```python
from build123d import *

# Parameters (mm, degrees)
SKETCH1_W           = 128
SKETCH1_H           = 73
SKETCH1_W_2         = 120
SKETCH1_H_2         = 65
BOSS_EXTRUDE1_DEPTH = 41
SKETCH1_3_W         = 128
SKETCH1_3_H         = 73
BOSS_EXTRUDE2_DEPTH = 4
SKETCH3_R           = 10.16
CUT_EXTRUDE1_DEPTH  = 4
SKETCH5_W           = 6
SKETCH5_H           = 65
BOSS_EXTRUDE3_DEPTH = 32
BOSS_EXTRUDE4_DEPTH = 32
CUT_EXTRUDE2_DEPTH  = 10


with BuildPart() as part:
    # Sketch1 → Boss-Extrude1 (new body)
    with BuildSketch(Plane(origin=(0, 0, 0), x_dir=(1, 0, 0), z_dir=(0, 1, 0))):
        Rectangle(SKETCH1_W, SKETCH1_H)
        Rectangle(SKETCH1_W_2, SKETCH1_H_2, mode=Mode.SUBTRACT)
    extrude(amount=BOSS_EXTRUDE1_DEPTH)

    # Sketch1<3> → Boss-Extrude2 (add)
    with BuildSketch(Plane(origin=(0, 0, 0), x_dir=(1, 0, 0), z_dir=(0, 1, 0))):
        Rectangle(SKETCH1_3_W, SKETCH1_3_H)
    extrude(amount=-BOSS_EXTRUDE2_DEPTH)

    # Sketch3 → Cut-Extrude1 (cut)
    with BuildSketch(Plane.XY.offset(36.5)):
        with Locations((-44, 21)):
            Circle(SKETCH3_R)
    extrude(amount=-CUT_EXTRUDE1_DEPTH, mode=Mode.SUBTRACT)

    # Sketch5 → Boss-Extrude3 (add)
    with BuildSketch(Plane(origin=(0, 0, 0), x_dir=(1, 0, 0), z_dir=(0, 1, 0))):
        with Locations((-11.5, 0)):
            Rectangle(SKETCH5_W, SKETCH5_H)
    extrude(amount=BOSS_EXTRUDE3_DEPTH)

    # Sketch8 → Boss-Extrude4 (add)
    with BuildSketch(Plane(origin=(0, 0, 0), x_dir=(1, 0, 0), z_dir=(0, 1, 0))):
        Polygon((-14.5, 32.5), (-22, 32.5), (-22, 21.3), (-19.5, 21.3), (-19.5, 26.3), (-14.5, 26.3), align=None)
        Polygon((-14.5, -26.3), (-14.5, -32.5), (-22, -32.5), (-22, -21.3), (-19.5, -21.3), (-19.5, -26.3), align=None)
    extrude(amount=BOSS_EXTRUDE4_DEPTH)

    # Sketch4 → Cut-Extrude2 (cut)
    with BuildSketch(Plane.ZY.offset(64)):
        with BuildLine():
            Line((10, 14.5), (-10, 14.5))
            ThreePointArc((-10, 14.5), (-14, 18.5), (-10, 22.5))
            Line((-10, 22.5), (10, 22.5))
            ThreePointArc((10, 22.5), (14, 18.5), (10, 14.5))
        make_face()
    extrude(amount=-CUT_EXTRUDE2_DEPTH, mode=Mode.SUBTRACT)


solid = part.part
```
Geometry: final body of the model. Coordinates: model frame, mm. A direction names the side the tool comes from. Coordinates: 2 decimals unless noted, no trailing zeros. Order: outer loops, then holes, each group sorted by start corner. A loop starts at its lowest first (then second) coordinate and runs counter-clockwise, first axis right, second up. Notation, with made-up numbers: (-36.5, -4) - (-24.5, -4) arc R22 ccw to (-24.5, 24) - close; hole circle Ø6 at (0, 1.25). An arc over 180 degrees is marked (long way). Write each question's results on one line, items separated by ' | '.
1) Section A-A, the plane y = 18.5. Return loops of the section in (x, z), plus the area to 3 significant figures.
Results list:
outline: (-64, -36.5) - (64, -36.5) - (64, 36.5) - (-34.15, 36.5) - (-34.15, 32.5) - (-22, 32.5) - (-22, 21.3) - (-19.5, 21.3) - (-19.5, 26.3) - (-14.5, 26.3) - (-14.5, -26.3) - (-19.5, -26.3) - (-19.5, -21.3) - (-22, -21.3) - (-22, -32.5) - (-60, -32.5) - (-60, -14) - (-64, -14) - close; (-64, 14) - (-60, 14) - (-60, 32.5) - (-53.85, 32.5) - (-53.85, 36.5) - (-64, 36.5) - close; hole (-8.5, -32.5) - (60, -32.5) - (60, 32.5) - (-8.5, 32.5) - close | area: 1,860 mm^2
2) Set-up query: faces 5 (the flat face through (-22, 16, 27)), 6 (the flat face through (-62, 22.5, 0)), 7 (the flat face through (-64, 24, 1)). Return all of +Z, -Z, +X, -X, +Y, -Y with unobstructed straight access to the full face (end or side cutting, diameter ignored); none if empty.
Results list:
face 5: +Y | face 6: -X | face 7: +Z, -Z, -X, +Y, -Y
3) Line query: line 1 (X direction, y = 9, z = -28); line 2 (X direction, y = 5, z = -8); line 3 (Z direction, x = 1, y = 27). Output: solid intervals per line, ascending. Write a range as from..to.
Results list:
line 1: -64..-60, -22..-8.5, 60..64 | line 2: -64..-60, -14.5..-8.5, 60..64 | line 3: -36.5..-32.5, 32.5..36.5
4) Section D-D, the plane y = 4.5. Return loops of the section in (x, z).
Results list:
outline: (-64, -36.5) - (64, -36.5) - (64, 36.5) - (-64, 36.5) - close; hole (-60, -32.5) - (-22, -32.5) - (-22, -21.3) - (-19.5, -21.3) - (-19.5, -26.3) - (-14.5, -26.3) - (-14.5, 26.3) - (-19.5, 26.3) - (-19.5, 21.3) - (-22, 21.3) - (-22, 32.5) - (-60, 32.5) - close; hole (-8.5, -32.5) - (60, -32.5) - (60, 32.5) - (-8.5, 32.5) - close
5) Section C-C, the plane z = -16. Return loops of the section in (x, y), plus the area to 3 significant figures.
Results list:
outline: (-64, -4) - (64, -4) - (64, 41) - (60, 41) - (60, 0) - (-8.5, 0) - (-8.5, 32) - (-14.5, 32) - (-14.5, 0) - (-60, 0) - (-60, 41) - (-64, 41) - close | area: 1,030 mm^2
6) Pin query (flat end, axial travel): pin 1 (3 mm diameter, centred on x = -0.5, z = 11.5, fed in from +Y); pin 2 (18.5 mm diameter, centred on x = -44, y = 21, fed in from +Z). Return the tip coordinate at first contact, or that it passes through.
Results list:
pin 1: y = 0 | pin 2: z = -32.5
7) Section B-B, the plane z = -5. Return loops of the section in (x, y), plus the area to 3 significant figures.
Results list:
outline: (-64, -4) - (64, -4) - (64, 41) - (60, 41) - (60, 0) - (-8.5, 0) - (-8.5, 32) - (-14.5, 32) - (-14.5, 0) - (-60, 0) - (-60, 14.5) - (-64, 14.5) - close; (-64, 22.5) - (-60, 22.5) - (-60, 41) - (-64, 41) - close | area: 1,000 mm^2
8) Pull-direction query (Y, two-part tool) for faces 1 (the flat face through (25, 0, 0)), 2 (the flat face through (-8.5, 16, 0)), 3 (the cylindrical face through (-62, 18.6, 14)), 4 (the flat face through (-62, 14.5, 0)); classes: pulls with the +Y half, pulls with the -Y half, needs draft (parallel to the pull), parting line crosses it, or undercut.
Results list:
face 1: pulls with the +Y half | face 2: needs draft | face 3: undercut | face 4: undercut
